Solid Edge part; units mm, degrees
sketch "Sketch1" plane through (0, 0, 0) normal (0, 0, 1) x (1, 0, 0)
  line L0 (1077.6266, -622.6959) -> (483.7062, -279.7959)
  line L1 (0.4572, -1244.6) -> (0.4572, -558.7998)
  line L2 (0.4572, -1244.6) -> (0.4572, -1930.3999)
  line L3 (1077.6266, -622.6959) -> (1671.5468, -965.5959)
  arc A0 (483.7062, -279.7959) -> (0.4572, -558.7998) centre (0, 0) cw
  arc A1 (1671.5468, -965.5959) -> (0.4572, -1930.3999) centre (0, 0) cw
  circle A2 centre (622.3, -1077.8552) radius 571.5
extrude "Protrusion1" add sketch "Sketch1" along normal blind 25.4
Design review of the part built by this model. Coordinates are the model's own, in mm. Give positions to 0.01 mm unless a question says otherwise; leave off trailing zeros. Write each loop counter-clockwise with the first axis right and the second up, starting at its lowest first coordinate (ties: lowest second). Pieces come first, ordered by that corner, then holes. Notation, with made-up numbers: (21.25, 32.25) -> (40.25, 32.25) arc R31 cw to (40.25, 57.25) -> close; hole circle Ø10 at (42.5, -2.5). An arc over 180 degrees is marked (long way). Answer in a Markdown table with one row per item.
(1) Consider section C-C (z = 10.25). State the section outline as (x, y) points.
Results:
| item | result |
|---|---|
| outline | (0.46, -1930.4) arc R1930.4 ccw to (1671.55, -965.6) -> (1077.63, -622.7) -> (483.71, -279.8) arc R558.8 cw to (0.46, -558.8) -> close; hole circle Ø1143 at (622.3, -1077.86) |
(2) To check wall thickness, follow probe 1 along Y at (x, z) = (622.3, 8.75); probe 2 along Y at (x, z) = (594, 9.75); probe 3 along X at (y, z) = (-931, 8.75). State the ranges of each line that lie inside material, in increasing order.
Results:
| item | result |
|---|---|
| probe 1 | -1827.34 to -1649.36, -506.36 to -359.81 |
| probe 2 | -1836.74 to -1648.65, -507.06 to -343.47 |
| probe 3 | 0.46 to 69.99, 1174.61 to 1611.62 |
(3) Consider section A-A (y = -590.5). State the section outline as (x, z) points.
Results:
| item | result |
|---|---|
| outline | (0.46, 0) -> (323.81, 0) -> (323.81, 25.4) -> (0.46, 25.4) -> close; (920.79, 0) -> (1021.86, 0) -> (1021.86, 25.4) -> (920.79, 25.4) -> close |
(4) Mouldability with a two-part tool opening along Y and no side actions: class faces 1 (the cylindrical face through (977.42, -1664.66, 12.52)), 2 (the flat face through (708, -1651, 0)), 3 (the cylindrical face through (1167.41, -1249.52, 12.52)) as +Y half, -Y half, draft (parallel to the pull), parting line (faces both ways), or undercut.
Results:
| item | result |
|---|---|
| face 1 | -Y half |
| face 2 | draft |
| face 3 | undercut |
(5) Consider section B-B (x = 166.5). State the section outline as (y, z) points.
Results:
| item | result |
|---|---|
| outline | (-1923.21, 0) -> (-1422.61, 0) -> (-1422.61, 25.4) -> (-1923.21, 25.4) -> close; (-733.1, 0) -> (-533.42, 0) -> (-533.42, 25.4) -> (-733.1, 25.4) -> close |
(6) Clearance check with flat-ended pins moving along their axes: pin 1 (4 mm diameter, centred on y = -593, z = 17.5, fed in from +X); pin 2 (1.5 mm diameter, centred on x = 1062.5, z = 16, fed in from +Y); pin 3 (12 mm diameter, centred on x = 497.5, z = 18.5, fed in from -Y). State where each tip first meets the part, or that it passes through.
Results:
| item | result |
|---|---|
| pin 1 | x = 1029.66 |
| pin 2 | y = -613.53 |
| pin 3 | y = -1866.78 |
(7) Consider section D-D (y = -1830). State the section outline as (x, z) points.
Results:
| item | result |
|---|---|
| outline | (0.46, 0) -> (614.45, 0) -> (614.45, 25.4) -> (0.46, 25.4) -> close |
